from build123d import *

# Parameters (mm, degrees)
F1_DEPTH = 100
F2_R     = 17.6104125338
F3_DEPTH = 100.001
F4_R     = 10
F5_DEPTH = 90.001


with BuildPart() as f1:
    # F0 (on Top) → F1 (new body)
    with BuildSketch(Plane.XY):
        with BuildLine():
            Line((0, 0), (-45, 0))
            ThreePointArc((-45, 0), (0, -45), (45, 0))
            ThreePointArc((45, 0), (23.4232921921, 38.4232921921), (-20.6155281281, 40))
            Line((-20.6155281281, 40), (0, 40))
            Line((0, 40), (0, 0))
        make_face()
        with BuildLine():
            Line((-45, 40), (-45, 0))
            ThreePointArc((-45, 0), (-38.4232921921, 23.4232921921), (-20.6155281281, 40))
            Line((-20.6155281281, 40), (-45, 40))
        make_face()
        with BuildLine():
            ThreePointArc((-20.6155281281, 40), (-38.4232921921, 23.4232921921), (-45, 0))
            Line((-45, 0), (0, 0))
            Line((0, 0), (0, 40))
            Line((0, 40), (-20.6155281281, 40))
        make_face()
    extrude(amount=F1_DEPTH)

    # F2 (on face) → F3 (cut, through all)
    with BuildSketch(Plane.XY.offset(100)):
        with Locations((5.4660397582, 20.4941760749)):
            Circle(F2_R)
    extrude(amount=-F3_DEPTH, mode=Mode.SUBTRACT)

    # F4 (on face) → F5 (cut, through all)
    with BuildSketch(Plane(origin=(-45, 0, 0), x_dir=(0, -1, 0), z_dir=(-1, 0, 0))):
        with Locations((-15, 30)):
            Circle(F4_R)
    extrude(amount=-F5_DEPTH, mode=Mode.SUBTRACT)


solid = f1.part
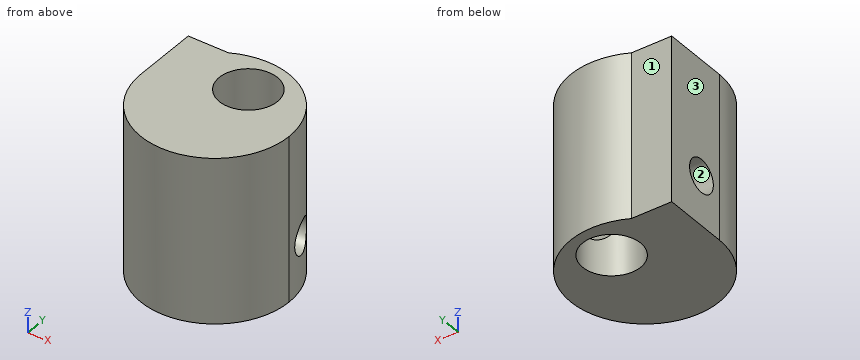
Input: part model. Units: mm. Frame: model coordinates. Face numbers are marked on the shaded views. Give positions to 0.01 mm unless a question says otherwise; leave off trailing zeros. Write each loop counter-clockwise with the first axis right and the second up, starting at its lowest first coordinate (ties: lowest second). Pieces come first, ordered by that corner, then holes.
Q1. Material intervals for probe 1 along Z at (x, y) = (-23, 15); probe 2 along X at (y, z) = (-1.5, 34) (3 decimals); probe 3 along Y at (x, z) = (21.5, 78), sorted ascending.
Q2. Section B-B, the plane z = 30. Output: boundary loops of the cut face in (x, y).
Q3. Section D-D, the plane x = 27.5. Output: boundary loops of the cut face in (y, z), plus the area to 3 significant figures.
Q4. Pull-direction query (Y, two-part tool) for the marked faces 1, 2 and 3; classes: pulls with the +Y half, pulls with the -Y half, needs draft (parallel to the pull), parting line crosses it, or undercut.
Q5. Section C-C, the plane x = 0. Output: boundary loops of the cut face in (y, z), plus the area to 3 significant figures.
Q6. Section A-A, the plane y = 15. Output: boundary loops of the cut face in (x, z), plus the area to 3 significant figures.
Q7. First-contact query: P1, Ø8, axis at x = -17, z = 25, coming from the -Y side; P2, Ø18, axis at y = 15, z = 30, coming from the +X side; P3, Ø10, axis at y = -13, z = 22.5, coming from the +X side; P4, Ø6, axis at x = -31, z = 51.5, coming from the +Y side. Flat tips, straight axial feed; report the tip coordinate or a pass-through.
Filled in:
1. probe 1: z = 0 to 20, 40 to 100
1. probe 2: x = -44.975 to 44.975
1. probe 3: y = -39.53 to 13.21, 27.78 to 39.53
2. outline: (-45, 0) arc R45 ccw (long way) to (44.72, 5) - (13.84, 5) arc R17.61 cw to (-2.9, 5) - (-45, 5) - close; (-45, 25) - (-11.56, 25) arc R17.61 cw to (22.49, 25) - (37.42, 25) arc R45 ccw to (-20.62, 40) - (-45, 40) - close
3. outline: (-35.62, 0) - (35.62, 0) - (35.62, 100) - (-35.62, 100) - close; hole circle Ø20 at (15, 30)
3. area: 6,810 mm2
4. face 1: pulls with the +Y half
4. face 2: undercut
4. face 3: needs draft
5. outline: (-45, 0) - (3.75, 0) - (3.75, 100) - (-45, 100) - close; (37.23, 0) - (45, 0) - (45, 100) - (37.23, 100) - close
5. area: 5,650 mm2
6. outline: (-45, 0) - (-11.27, 0) - (-11.27, 20) - (-45, 20) - close; (-45, 40) - (-11.27, 40) - (-11.27, 100) - (-45, 100) - close; (22.2, 0) - (42.43, 0) - (42.43, 20) - (22.2, 20) - close; (22.2, 40) - (42.43, 40) - (42.43, 100) - (22.2, 100) - close
6. area: 4,320 mm2
7. P1: stops at y = -43.08
7. P2: passes through
7. P3: stops at x = 44.28
7. P4: stops at y = 40
